Can you work these out from the model? Positions are in its coordinate system, mm. Face numbers are marked on the shaded views. A direction names the side the tool comes from. Give positions to 0.01 mm unless a question says otherwise; leave off trailing zeros. Loops run counter-clockwise (first coordinate to the right, second up) from the corner with the lowest first, then second, coordinate; pieces in that order, holes last. Notation, with made-up numbers: M 54,20 L 113,20 A22 ccw 113,34 Z; hole C -36,78 d6. An arc over 180 degrees is marked long. Answer as a JSON object with one key per item and string values.
```python
from build123d import *

# Parameters (mm, degrees)
SKETCH1_W           = 60
SKETCH1_H           = 50
BOSS_EXTRUDE1_DEPTH = 10
CUT_REVOLVE1_DEPTH  = 30


# Read off the part's stored shape, not the designer's step: Cut-Revolve1
with BuildPart() as part:
    # Sketch1 → Boss-Extrude1 (new, symmetric)
    with BuildSketch(Plane.XY):
        with Locations((0, 15)):
            Rectangle(SKETCH1_W, SKETCH1_H)
    extrude(amount=BOSS_EXTRUDE1_DEPTH, both=True)

    # Cut-Revolve1 outline → Cut-Revolve1 (cut)
    with BuildSketch(Plane(origin=(0, 0, 0), x_dir=(1, 0, 0), z_dir=(0, 1, 0))):
        with BuildLine():
            ThreePointArc((17.320508076, -10), (20, 0), (17.320508076, 10))
            Line((17.320508076, 10), (5.773502692, 10))
            Line((5.773502692, 10), (2.5, 4.330127019))
            ThreePointArc((2.5, 4.330127019), (5, 0), (2.5, -4.330127019))
            Line((2.5, -4.330127019), (5.773502692, -10))
            Line((5.773502692, -10), (17.320508076, -10))
        make_face()
    extrude(amount=CUT_REVOLVE1_DEPTH, mode=Mode.SUBTRACT)


solid = part.part
```
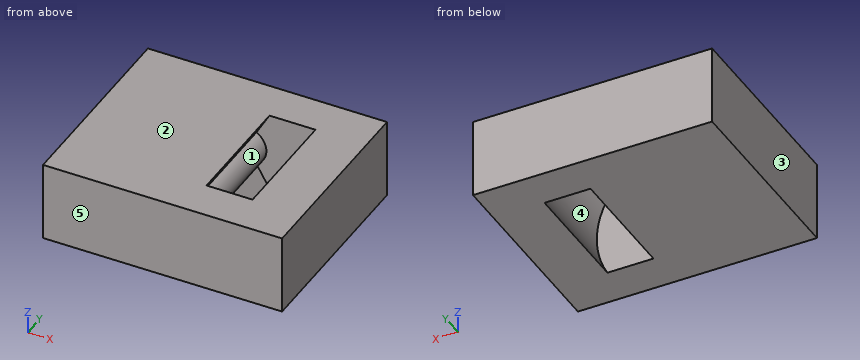
1) Suppose I cut it at C-C, the plane x = 4. Write out the boundary of the cut face in (y, z).
Answer list:
{"outline": "M -10,-10 L 40,-10 L 40,10 L -10,10 Z; hole M 0,-6.93 L 30,-6.93 L 30,-3 L 0,-3 Z; hole M 0,3 L 30,3 L 30,6.93 L 0,6.93 Z"}
2) Please list where these lines run through material, in increasing order: line 1 along Y through (x, z) = (8.5, -9); line 2 along X through (y, z) = (11, 7.5); line 3 along X through (y, z) = (3.5, -0.25). Write a range as from..to.
Answer list:
{"line 1": "-10..0, 30..40", "line 2": "-30..4.33, 18.54..30", "line 3": "-30..4.99, 20..30"}
3) For the marked faces 4 and 5, which set-ups out of +Z, -Z, +X, -X, +Y, -Y let a thin tool reach every point of the face, with its end or its side?
Answer list:
{"face 4": "none", "face 5": "+Z, -Z, +X, -X, -Y"}
4) Suppose I cut it at A-A, the plane y = 25. Write out the boundary of the cut face in (x, z).
Answer list:
{"outline": "M -30,-10 L 5.77,-10 L 2.5,-4.33 A5 ccw 2.5,4.33 L 5.77,10 L -30,10 Z; M 17.32,-10 L 30,-10 L 30,10 L 17.32,10 A20 cw Z"}
5) If we mould it in two halves opening along Z, with no side actions, what happens to the marked faces 1, 2 and 3? For each: +Z half, -Z half, draft (parallel to the pull), parting line (faces both ways), or undercut.
Answer list:
{"face 1": "undercut", "face 2": "+Z half", "face 3": "draft"}
6) Suppose I cut it at B-B, the plane z = -5.5. Write out the boundary of the cut face in (x, y), and give its area (3 significant figures).
Answer list:
{"outline": "M -30,-10 L 30,-10 L 30,40 L -30,40 Z; hole M 3.18,0 L 19.23,0 L 19.23,30 L 3.18,30 Z", "area": "2,520 mm^2"}
7) Suppose I cut it at D-D, the plane z = 3.5. Write out the boundary of the cut face in (x, y).
Answer list:
{"outline": "M -30,-10 L 30,-10 L 30,40 L -30,40 Z; hole M 3.57,0 L 19.69,0 L 19.69,30 L 3.57,30 Z"}
